Input: part model. Units: mm. Frame: model coordinates. A direction names the side the tool comes from. Coordinates: 2 decimals unless noted, no trailing zeros. Loops run counter-clockwise (first coordinate to the right, second up) from the corner with the lowest first, then second, coordinate; pieces in that order, holes last.
```python
from build123d import *

# Parameters (mm, degrees)
SKETCH_288_R           = 30.65
SKETCH_288_R_2         = 2.25
EXTRUDE_1509_DEPTH     = 10
SKETCH_1_3_R           = 3.55
CUT_EXTRUDE_1553_DEPTH = 5
SKETCH_1_5_W           = 10.5
SKETCH_1_5_H           = 30
EXTRUDE_2_DEPTH        = 12
CUT_EXTRUDE_2473_REACH = 50.706
SKETCH_2180_R          = 2.15


with BuildPart() as part:
    # Sketch 288 → Extrude 1509 (new body)
    with BuildSketch(Plane.XY):
        Circle(SKETCH_288_R)
        with Locations((24.65, 0)):
            Circle(SKETCH_288_R_2, mode=Mode.SUBTRACT)
        with Locations((-12.325, -21.347526203)):
            Circle(SKETCH_288_R_2, mode=Mode.SUBTRACT)
        with Locations((-12.325, 21.347526203)):
            Circle(SKETCH_288_R_2, mode=Mode.SUBTRACT)
    extrude(amount=EXTRUDE_1509_DEPTH)

    # Sketch 1_3 → Cut-Extrude 1553 (cut)
    with BuildSketch(Plane.XY):
        with Locations((24.65, 0)):
            Circle(SKETCH_1_3_R)
        with Locations((-12.325, -21.347526203)):
            Circle(SKETCH_1_3_R)
        with Locations((-12.325, 21.347526203)):
            Circle(SKETCH_1_3_R)
    extrude(amount=CUT_EXTRUDE_1553_DEPTH, mode=Mode.SUBTRACT)

    # Sketch 1_5 → Extrude 2 (add)
    with BuildSketch(Plane.XY):
        Rectangle(SKETCH_1_5_W, SKETCH_1_5_H)
    extrude(amount=-EXTRUDE_2_DEPTH)

    # Sketch 2180 → Cut-Extrude 2473 (cut, up to next)
    with BuildSketch(Plane.ZY.offset(5.25), mode=Mode.PRIVATE) as cut_extrude_2473_sk1:
        with Locations((-5, 7.5)):
            Circle(SKETCH_2180_R)
    cut_extrude_2473_tool1 = extrude(cut_extrude_2473_sk1.sketch, amount=-CUT_EXTRUDE_2473_REACH, mode=Mode.PRIVATE) & part.part
    # Sketch 2180 → Cut-Extrude 2473 (cut, up to next)
    with BuildSketch(Plane.ZY.offset(5.25), mode=Mode.PRIVATE) as cut_extrude_2473_sk2:
        with Locations((-5, -7.5)):
            Circle(SKETCH_2180_R)
    cut_extrude_2473_tool2 = extrude(cut_extrude_2473_sk2.sketch, amount=-CUT_EXTRUDE_2473_REACH, mode=Mode.PRIVATE) & part.part
    add(cut_extrude_2473_tool1.solids().sort_by_distance((-5.25, 7.5, -5))[0], mode=Mode.SUBTRACT)
    add(cut_extrude_2473_tool2.solids().sort_by_distance((-5.25, -7.5, -5))[0], mode=Mode.SUBTRACT)


solid = part.part
```
Item 1: Line query: L1, parallel to Y at x = -0.75, z = -5; L2, parallel to Z at x = -14.5, y = 14; L3, parallel to X at y = 14, z = -1. Output: solid intervals per line, ascending.
Result:
L1: y = -15 to -9.65, -5.35 to 5.35, 9.65 to 15
L2: z = 0 to 10
L3: x = -5.25 to 5.25
Item 2: Reachability of faces 1 (the face through (-0.074, -6.047, -6.585)), 2 (the face through (-13.095, -24.813, 2.465)), 3 (the face through (5.25, 0, -6)), 4 (the face through (-5.25, 0, -6)) from +Z, -Z, +X, -X, +Y, -Y: full face, straight path, thin tool, end or side. Return the list, or none.
Result:
face 1: +X, -X
face 2: -Z
face 3: -Z, +X, +Y, -Y
face 4: -Z, -X, +Y, -Y
Item 3: Section query D-D (y = -11). Output: boundary loops of the cut face in (x, z), then the cut area to 3 significant figures.
Result:
outline: (-28.61, 0) - (-5.25, 0) - (-5.25, -12) - (5.25, -12) - (5.25, 0) - (28.61, 0) - (28.61, 10) - (-28.61, 10) - close
area: 698 mm2
Item 4: Section query A-A (z = -5). Output: boundary loops of the cut face in (x, y), then the cut area to 3 significant figures.
Result:
outline: (-5.25, -15) - (5.25, -15) - (5.25, -9.65) - (-5.25, -9.65) - close; (-5.25, -5.35) - (5.25, -5.35) - (5.25, 5.35) - (-5.25, 5.35) - close; (-5.25, 9.65) - (5.25, 9.65) - (5.25, 15) - (-5.25, 15) - close
area: 225 mm2
Item 5: Section query B-B (x = 0). Output: boundary loops of the cut face in (y, z), then the cut area to 3 significant figures.
Result:
outline: (-30.65, 0) - (-15, 0) - (-15, -12) - (15, -12) - (15, 0) - (30.65, 0) - (30.65, 10) - (-30.65, 10) - close; hole circle Ø4.3 at (-7.5, -5); hole circle Ø4.3 at (7.5, -5)
area: 944 mm2
Item 6: Contact query for flat-ended pins moving along their axis: P1, Ø4, axis at y = 7.5, z = -5, coming from the +X side; P2, Ø1, axis at y = -12.5, z = -1.5, coming from the -X side; P3, Ø12, axis at x = -6, z = 1, coming from the +Y side; P4, Ø3.5, axis at x = -13, y = -20.5, coming from the -Z side. Output: stop coordinate, or through.
Result:
P1: passes through
P2: stops at x = -5.25
P3: stops at y = 30.65
P4: stops at z = 5
Item 7: Section query C-C (y = 0). Output: boundary loops of the cut face in (x, z), then the cut area to 3 significant figures.
Result:
outline: (-30.65, 0) - (-5.25, 0) - (-5.25, -12) - (5.25, -12) - (5.25, 0) - (21.1, 0) - (21.1, 5) - (22.4, 5) - (22.4, 10) - (-30.65, 10) - close; (26.9, 5) - (28.2, 5) - (28.2, 0) - (30.65, 0) - (30.65, 10) - (26.9, 10) - close
area: 681 mm2
Item 8: Mould query, pull axis Y, two halves, no side actions, for faces 5 (the face through (0, 15, -6)), 6 (the face through (-13.09, 17.88, 2.46)), 7 (the face through (0, -15, -6)). Classes: +Y half, -Y half, draft (parallel to the pull), parting line (faces both ways), or undercut.
Result:
face 5: +Y half
face 6: undercut
face 7: -Y half
